```python
from build123d import *

# Parameters (mm, degrees)
AUFSATZ_LINEAR_AUSTRAGEN1_DEPTH = 6
SKIZZE4_R                       = 1
SCHNITT_LINEAR_AUSTRAGEN1_DEPTH = 3
SCHNITT_LINEAR_AUSTRAGEN2_DEPTH = 3.8
VERRUNDUNG1_R                   = 0.4
SCHNITT_LINEAR_AUSTRAGEN6_DEPTH = 6
AUFSATZ_LINEAR_AUSTRAGEN2_DEPTH = 3


with BuildPart() as part:
    # Skizze1 → Aufsatz-Linear austragen1 (new body)
    with BuildSketch(Plane.XY):
        Polygon((0, 0), (7.5, 0), (7.5, 3), (31.5, 3), (31.5, 0), (39, 0), (39, 1), (33.5, 5), (5.5, 5), (0, 1), align=None)
    extrude(amount=AUFSATZ_LINEAR_AUSTRAGEN1_DEPTH)

    # Skizze4 → Schnitt-Linear austragen1 (cut)
    with BuildSketch(Plane.XZ):
        with Locations(Location((36.25, 3, 0), (0, 0, 270))):
            Circle(SKIZZE4_R)
    schnitt_linear_austragen1 = extrude(amount=-SCHNITT_LINEAR_AUSTRAGEN1_DEPTH, mode=Mode.SUBTRACT)

    # Skizze5 → Schnitt-Linear austragen2 (cut)
    with BuildSketch(Plane(origin=(0, 5, 0), x_dir=(-1, 0, 0), z_dir=(0, -1, 0))):
        with BuildLine():
            Line((-36.25, -5.2), (-39, -5.2))
            Line((-39, -5.2), (-39, -0.8))
            Line((-39, -0.8), (-36.25, -0.8))
            ThreePointArc((-36.25, -0.8), (-34.05, -3), (-36.25, -5.2))
        make_face()
    schnitt_linear_austragen2 = extrude(amount=SCHNITT_LINEAR_AUSTRAGEN2_DEPTH, mode=Mode.SUBTRACT)

    # Spiegeln1: Schnitt-Linear austragen1, Schnitt-Linear austragen2 across plane
    add(schnitt_linear_austragen1.mirror(Plane.ZY.offset(-19.5)), mode=Mode.SUBTRACT)
    add(schnitt_linear_austragen2.mirror(Plane.ZY.offset(-19.5)), mode=Mode.SUBTRACT)

    # Verrundung1
    verrundung1_edges = [part.edges().sort_by_distance(p)[0] for p in [
        (36.25, 3, 0),
        (36.25, 3, 6),
        (2.75, 3, 6),
        (2.75, 3, 0),
    ]]
    fillet(verrundung1_edges, radius=VERRUNDUNG1_R)

    # Skizze10 → Schnitt-Linear austragen6 (cut)
    with BuildSketch(Plane(origin=(0, 5, 0), x_dir=(-1, 0, 0), z_dir=(0, -1, 0))):
        with BuildLine():
            Line((-36, 0), (-39, 0))
            Line((-39, 0), (-39.338530881, 0))
            Line((-39.338530881, 0), (-39.338530881, -6))
            Line((-39.338530881, -6), (-36, -6))
            ThreePointArc((-36, -6), (-39, -3), (-36, 0))
        make_face()
    schnitt_linear_austragen6 = extrude(amount=SCHNITT_LINEAR_AUSTRAGEN6_DEPTH, mode=Mode.SUBTRACT)

    # Spiegeln2: Schnitt-Linear austragen6 across plane
    add(schnitt_linear_austragen6.mirror(Plane.ZY.offset(-19.5)), mode=Mode.SUBTRACT)

    # Skizze12 → Aufsatz-Linear austragen2 (add)
    with BuildSketch(Plane.XZ.offset(-3)):
        with BuildLine():
            Line((31.5, 1.75), (29.5, 1.75))
            ThreePointArc((29.5, 1.75), (28.25, 3), (29.5, 4.25))
            Line((29.5, 4.25), (31.5, 4.25))
            Line((31.5, 4.25), (31.5, 1.75))
        make_face()
    aufsatz_linear_austragen2 = extrude(amount=AUFSATZ_LINEAR_AUSTRAGEN2_DEPTH)

    # Spiegeln3: Aufsatz-Linear austragen2 across plane
    add(aufsatz_linear_austragen2.mirror(Plane.ZY.offset(-19.5)))


solid = part.part
```
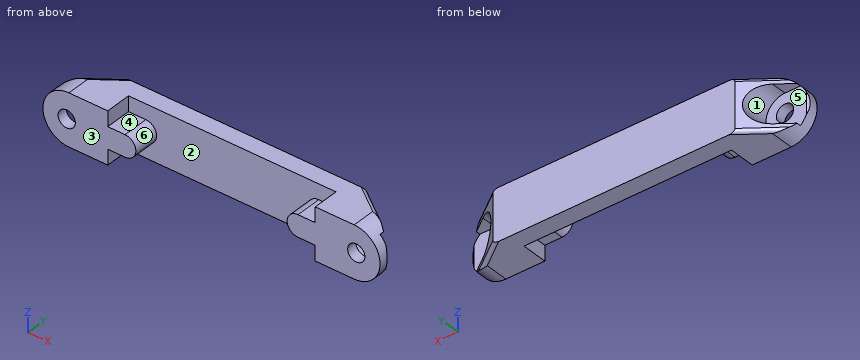
Can you work these out from the model? Positions are in its coordinate system, mm. Face numbers are marked on the shaded views. A direction names the side the tool comes from. Give positions to 0.01 mm unless a question says otherwise; leave off trailing zeros. Order: outer loops, then holes, each group sorted by start corner. A loop starts at its lowest first (then second) coordinate and runs counter-clockwise, first axis right, second up. Notation, with made-up numbers: M 86,16.5 L 115,16.5 A20 ccw 115,55.5 Z; hole C 34,1.25 d8. An arc over 180 degrees is marked long. Write item = value, one per line. Start each with the question number.
Q1. Will these pins go through, and if not, where does the flat tip stop? pin 1 Ø1.6 at (x, y) = (8.5, 1) entering from +Z; pin 2 Ø1.9 at (y, z) = (2, 5) entering from -X; pin 3 Ø3 at (y, z) = (1.5, 4.5) entering from -X; pin 4 Ø1.4 at (x, y) = (1.5, 2.5) entering from -Z.
Q2. Suppose I cut it at B-B (x = 18.5). Write out the boundary of the cut face in (y, z), plus the area to 3 significant figures.
Q3. For the marked faces 4, 5 and 6, which set-ups out of +Z, -Z, +X, -X, +Y, -Y let a thin tool reach every point of the face, with its end or its side?
Q4. We'd pull the mould along X, two halves only. Please class the marked faces 1, 2 and 3: pulls with the +X half, pulls with the -X half, needs draft (parallel to the pull), parting line crosses it, or undercut.
Q5. Suppose I cut it at A-A (z = 3). Write out the boundary of the cut face in (x, y) (3 decimals).
Q6. I need wall thicknesses on probe 1 along X at (y, z) = (0.65, 3); probe 2 along Z at (x, y) = (37, 0.7); probe 3 along Z at (x, y) = (2.75, 0.7). Which ranges of each line are inside material? Lowest first, please. Write a range as [from, to].
Check result:
q1.pin_1 = 4.25
q1.pin_2 = 0.39
q1.pin_3 = 0
q1.pin_4 = 0.11
q2.outline = M 3,0 L 5,0 L 5,6 L 3,6 Z
q2.area = 12.0 mm2
q3.face_4 = +Z, -Y
q3.face_5 = -X, +Y
q3.face_6 = -Y
q4.face_1 = pulls with the -X half
q4.face_2 = undercut
q4.face_3 = needs draft
q5.outline = M 0,0 L 1.75,0 L 1.75,1.2 L 0.275,1.2 L 0,1 Z; M 3.75,0 L 10.75,0 L 10.75,3 L 28.25,3 L 28.25,0 L 35.25,0 L 35.25,1.2 L 34.05,1.2 L 34.05,4.6 L 33.5,5 L 5.5,5 L 4.95,4.6 L 4.95,1.2 L 3.75,1.2 Z; M 37.25,0 L 39,0 L 39,1 L 38.725,1.2 L 37.25,1.2 Z
q6.probe_1 = [0, 1.75], [3.75, 10.75], [28.25, 35.25], [37.25, 39]
q6.probe_2 = [0.17, 2.34], [3.66, 5.83]
q6.probe_3 = [0.01, 2], [4, 5.99]
